Could you check a few things on this drawing? It's one solid part, dimensions in mm from its lowest x, y, z. A direction names the side the tool comes from. Coordinates: 2 decimals unless noted, no trailing zeros. Write each loop counter-clockwise with the first axis right and the second up, starting at its lowest first coordinate (ties: lowest second). Pieces come first, ordered by that corner, then holes. Notation, with made-up numbers: (37.25, -8.5) - (53.25, -8.5) arc R28 cw to (53.25, 9.5) - close; hole circle Ø9 at (-21.75, -9). An arc over 180 degrees is marked (long way). Use one line per item in the form item = value. Start each with the question number.
(1) If we section it at D-D on z = 4.5: Please give me the cut outline in (x, y).
(2) If I drill on probe 1 along X at (y, z) = (1.75, 1); probe 2 along X at (y, z) = (2.5, 6); probe 3 along Y at (x, z) = (2.25, 6), over which ranges is the centre line in solid material (lowest first)? Write a range as from..to.
(3) If we section it at A-A on y = 3.5: Please give me the cut outline in (x, z), then the cut area to 3 significant figures.
(4) If we section it at C-C on z = 1: Please give me the cut outline in (x, y).
(5) On a 3-axis mill with a long thin cutter (end or side, diameter ignored), from which of +Z, -Z, +X, -X, +Y, -Y can I reach the whole of each face in a straight line? I mean the marked faces 1 and 2. Say none if no direction works.
(6) For pin 1 Ø4 at (y, z) = (3.5, 7) entering from -X; pin 2 Ø1.5 at (x, y) = (5.5, 1.5) entering from +Z; pin 3 Ø1 at (x, z) = (4, 3.5) entering from -Y; pin 4 Ø1 at (y, z) = (4, 4) entering from +X, each with a flat end and sliding along its axis, tell me the tip position at first contact or that it passes through.
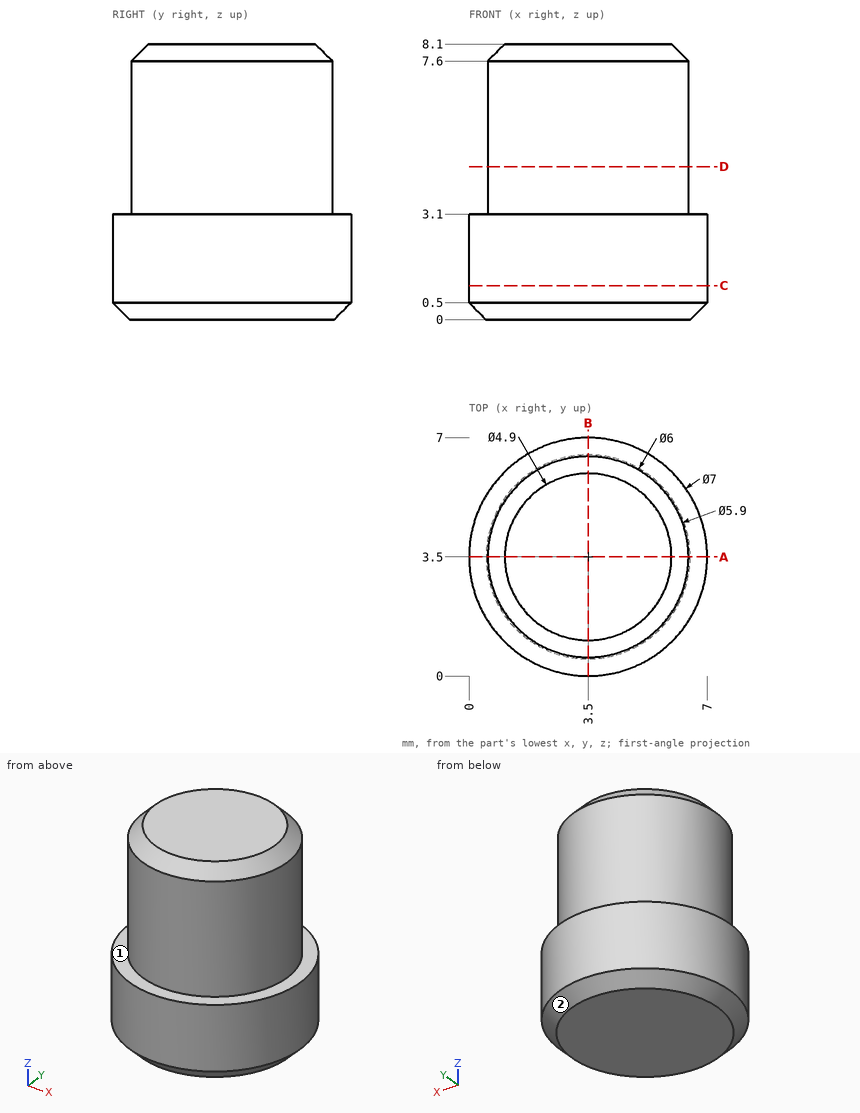
Reported:
q1.outline = circle Ø5.9 at (3.5, 3.5)
q2.probe_1 = 0.47..6.53
q2.probe_2 = 0.72..6.28
q2.probe_3 = 0.83..6.17
q3.outline = (0, 0.5) - (0.5, 0) - (6.5, 0) - (7, 0.5) - (7, 3.1) - (6.45, 3.1) - (6.45, 7.6) - (5.95, 8.1) - (1.05, 8.1) - (0.55, 7.6) - (0.55, 3.1) - (0, 3.1) - close
q3.area = 50.7 mm2
q4.outline = circle Ø7 at (3.5, 3.5)
q5.face_1 = +Z
q5.face_2 = -Z
q6.pin_1 = 0.55
q6.pin_2 = 8.1
q6.pin_3 = 0.01
q6.pin_4 = 6.45
